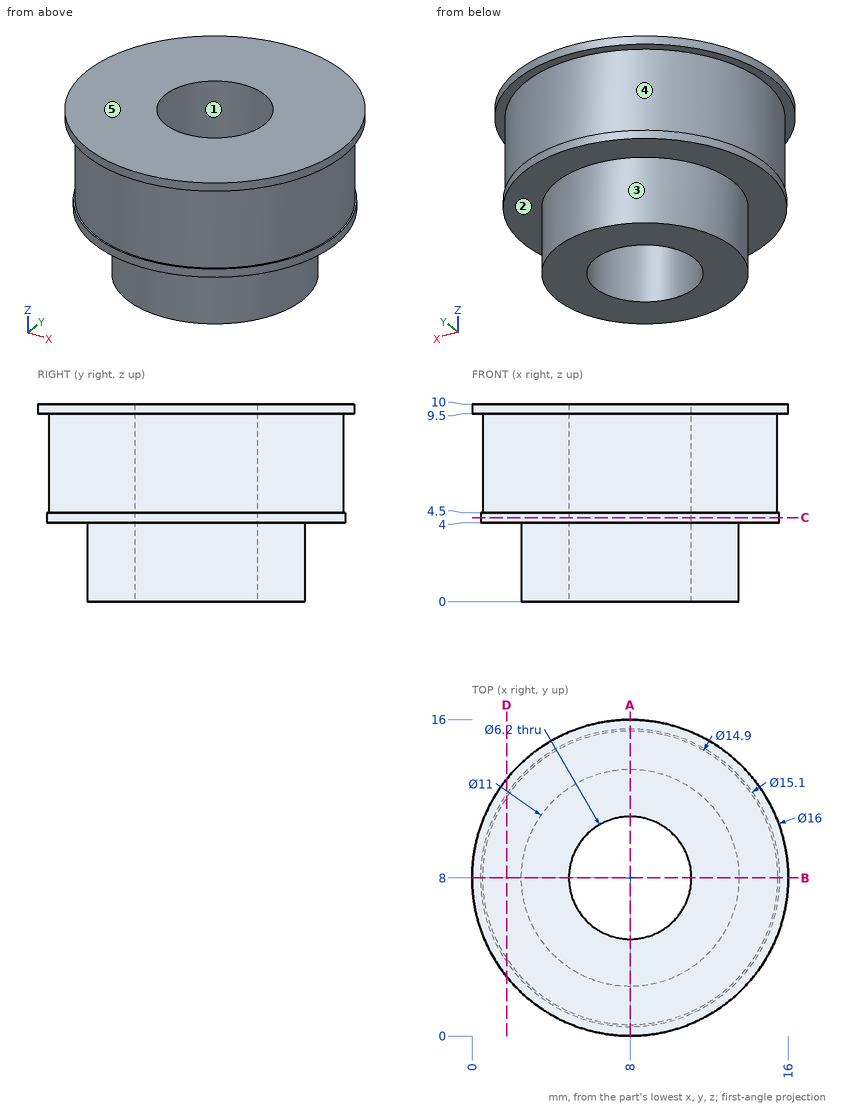
Answer from the drawing. Dimensions are ordinates in mm from the lowest x, y and z of the part. A direction names the side the tool comes from. Coordinates: 2 decimals unless noted, no trailing zeros. Order: outer loops, then holes, each group sorted by start corner. A loop starts at its lowest first (then second) coordinate and runs counter-clockwise, first axis right, second up. Notation, with made-up numbers: (16.5, 87) - (73.5, 87) arc R12 cw to (73.5, 105) - close; hole circle Ø10 at (2.25, -9). An arc over 180 degrees is marked (long way). Use one line per item in the form item = value.
(1) Section A-A, the plane x = 8 is taken. Give the vertices of the cut face in (y, z).
Computed values:
outline = (0, 9.5) - (0.55, 9.5) - (0.55, 4.5) - (0.45, 4.5) - (0.45, 4) - (2.5, 4) - (2.5, 0) - (4.9, 0) - (4.9, 10) - (0, 10) - close; (11.1, 0) - (13.5, 0) - (13.5, 4) - (15.55, 4) - (15.55, 4.5) - (15.45, 4.5) - (15.45, 9.5) - (16, 9.5) - (16, 10) - (11.1, 10) - close
(2) Given pin 1 Ø7 at (x, y) = (8, 8) entering from -Z; pin 2 Ø2 at (y, z) = (13.5, 1.5) entering from +X; pin 3 Ø4 at (y, z) = (4, 1.5) entering from +X; pin 4 Ø5 at (x, z) = (14, 6.5) entering from -Y, each flat-ended and moving along its own axis, determine where each tip first touches the part or whether it passes through.
Computed values:
pin_1 = 0
pin_2 = 11.16
pin_3 = 13.12
pin_4 = 1.42
(3) Which of the six approach directions +Z, -Z, +X, -X, +Y, -Y give full straight-line access (tool end or side, diameter ignored) to the marked faces 1 and 2?
Computed values:
face_1 = +Z, -Z
face_2 = -Z
(4) For a pull along Z with two mould halves and no side action, classify the marked faces 3, 4 and 5 as pulls with the +Z half, pulls with the -Z half, needs draft (parallel to the pull), parting line crosses it, or undercut.
Computed values:
face_3 = needs draft
face_4 = undercut
face_5 = pulls with the +Z half
(5) Section C-C, the plane z = 4.25 is taken. Give the vertices of the cut face in (x, y).
Computed values:
outline = circle Ø15.1 at (8, 8); hole circle Ø6.2 at (8, 8)
(6) Section D-D, the plane x = 1.75 is taken. Give the vertices of the cut face in (y, z).
Computed values:
outline = (3.01, 9.5) - (3.95, 9.5) - (3.95, 4.5) - (3.76, 4.5) - (3.76, 4) - (12.24, 4) - (12.24, 4.5) - (12.05, 4.5) - (12.05, 9.5) - (12.99, 9.5) - (12.99, 10) - (3.01, 10) - close
(7) Straight lines are drawn through the part: L1, parallel to Y at x = 8, z = 8; L2, parallel to Y at x = 8, z = 2; L3, parallel to Z at x = 13, y = 4.25. For each, find the intervals that lie inside material, in ascending order.
Computed values:
L1 = 0.55 to 4.9, 11.1 to 15.45
L2 = 2.5 to 4.9, 11.1 to 13.5
L3 = 4 to 10
